from build123d import *

# Parameters (mm, degrees)
SKETCH_W        = 61
SKETCH_H        = 50
PAD_DEPTH       = 40
SKETCH001_W     = 58
SKETCH001_H     = 47
POCKET_DEPTH    = 23
SKETCH002_W     = 56
SKETCH002_H     = 45
POCKET001_DEPTH = 16
SKETCH003_W     = 1
SKETCH003_H     = 45
PAD001_DEPTH    = 3
SKETCH004_W     = 4
SKETCH004_H     = 11
POCKET002_DEPTH = 5
SKETCH005_W     = 5.5
SKETCH005_H     = 15.5
POCKET003_DEPTH = 23
SKETCH006_W     = 59
SKETCH006_H     = 48
POCKET004_DEPTH = 1
SKETCH007_W     = 2.5
SKETCH007_H     = 3.5
POCKET005_DEPTH = 23
SKETCH009_W     = 10
SKETCH009_H     = 5
POCKET006_DEPTH = 5
PAD002_DEPTH    = 2
SKETCH011_W     = 8
SKETCH011_H     = 4.5
POCKET007_DEPTH = 5
SKETCH012_W     = 15.5
SKETCH012_H     = 6
POCKET008_DEPTH = 5
SKETCH013_W     = 9
SKETCH013_H     = 1
POCKET009_DEPTH = 3
SKETCH014_W     = 1
SKETCH014_H     = 4.5
POCKET010_DEPTH = 5
SKETCH015_W     = 9
SKETCH015_H     = 0.5
POCKET011_DEPTH = 5
SKETCH016_W     = 17.5
SKETCH016_H     = 1
POCKET012_DEPTH = 5
SKETCH017_W     = 2
SKETCH017_H     = 6
POCKET013_DEPTH = 5
SKETCH018_W     = 1
SKETCH018_H     = 11
POCKET014_DEPTH = 5
SKETCH019_W     = 12
SKETCH019_H     = 1.5
POCKET015_DEPTH = 5
SKETCH020_W     = 2
SKETCH020_H     = 5
POCKET016_DEPTH = 5
SKETCH021_R     = 2.692582
POCKET017_DEPTH = 5
SKETCH022_W     = 1
SKETCH022_H     = 45
PAD003_DEPTH    = 3
SKETCH023_W     = 41
SKETCH023_H     = 1
PAD004_DEPTH    = 3
SKETCH024_W     = 1
SKETCH024_H     = 45
POCKET018_DEPTH = 3


with BuildPart() as part:
    # Sketch → Pad (new body)
    with BuildSketch(Plane.XY):
        with Locations((30.5, 25)):
            Rectangle(SKETCH_W, SKETCH_H)
    extrude(amount=PAD_DEPTH)

    # Sketch001 (on Face6 of Pad) → Pocket (cut)
    with BuildSketch(Plane.XY.offset(40)):
        with Locations((30.5, 25)):
            Rectangle(SKETCH001_W, SKETCH001_H)
    extrude(amount=-POCKET_DEPTH, mode=Mode.SUBTRACT)

    # Sketch002 (on Face11 of Pocket) → Pocket001 (cut)
    with BuildSketch(Plane.XY.offset(17)):
        with Locations((30.5, 25)):
            Rectangle(SKETCH002_W, SKETCH002_H)
    extrude(amount=-POCKET001_DEPTH, mode=Mode.SUBTRACT)

    # Sketch003 (on Face16 of Pocket001) → Pad001 (join)
    with BuildSketch(Plane.XY.offset(1)):
        with Locations((45, 25)):
            Rectangle(SKETCH003_W, SKETCH003_H)
    extrude(amount=PAD001_DEPTH)

    # Sketch004 (on Face20 of Pad001) → Pocket002 (cut)
    with BuildSketch(Plane.XY.offset(1)):
        with Locations((5, 13)):
            Rectangle(SKETCH004_W, SKETCH004_H)
    extrude(amount=-POCKET002_DEPTH, mode=Mode.SUBTRACT)

    # Sketch005 (on Face5 of Pocket002) → Pocket003 (cut)
    with BuildSketch(Plane.XY.offset(40)):
        with Locations((58.25, 42.25)):
            Rectangle(SKETCH005_W, SKETCH005_H)
    extrude(amount=-POCKET003_DEPTH, mode=Mode.SUBTRACT)

    # Sketch006 (on Face5 of Pocket003) → Pocket004 (cut)
    with BuildSketch(Plane.XY.offset(40)):
        with Locations((30.5, 25)):
            Rectangle(SKETCH006_W, SKETCH006_H)
    extrude(amount=-POCKET004_DEPTH, mode=Mode.SUBTRACT)

    # Sketch007 (on Face5 of Pocket004) → Pocket005 (cut)
    with BuildSketch(Plane.XY.offset(40)):
        with Locations((59.75, 32.75)):
            Rectangle(SKETCH007_W, SKETCH007_H)
    extrude(amount=-POCKET005_DEPTH, mode=Mode.SUBTRACT)

    # Sketch009 (on Face1 of Pocket005) → Pocket006 (cut)
    with BuildSketch(Plane.XZ):
        with Locations((21, 23.5)):
            Rectangle(SKETCH009_W, SKETCH009_H)
    extrude(amount=-POCKET006_DEPTH, mode=Mode.SUBTRACT)

    # Sketch010 (on Face21 of Pocket006) → Pad002 (join)
    with BuildSketch(Plane.XY.offset(17)):
        Polygon((55.5, 50), (61, 50), (61, 31), (59.5, 31), (59.5, 48.5), (55.5, 48.5), align=None)
    extrude(amount=PAD002_DEPTH)

    # Sketch011 (on Face31 of Pad002) → Pocket007 (cut)
    with BuildSketch(Plane.YZ.offset(2.5)):
        with Locations((8, 9.75)):
            Rectangle(SKETCH011_W, SKETCH011_H)
    extrude(amount=-POCKET007_DEPTH, mode=Mode.SUBTRACT)

    # Sketch012 (on Face28 of Pocket007) → Pocket008 (cut)
    with BuildSketch(Plane.YZ.offset(2.5)):
        with Locations((29.25, 8)):
            Rectangle(SKETCH012_W, SKETCH012_H)
    extrude(amount=-POCKET008_DEPTH, mode=Mode.SUBTRACT)

    # Sketch013 (on Face2 of Pocket008) → Pocket009 (cut)
    with BuildSketch(Plane(origin=(0, 0, 0), x_dir=(0, -1, 0), z_dir=(-1, 0, 0))):
        with Locations((-8.5, 12.5)):
            Rectangle(SKETCH013_W, SKETCH013_H)
    extrude(amount=-POCKET009_DEPTH, mode=Mode.SUBTRACT)

    # Sketch014 (on Face2 of Pocket009) → Pocket010 (cut)
    with BuildSketch(Plane(origin=(0, 0, 0), x_dir=(0, -1, 0), z_dir=(-1, 0, 0))):
        with Locations((-12.5, 9.75)):
            Rectangle(SKETCH014_W, SKETCH014_H)
    extrude(amount=-POCKET010_DEPTH, mode=Mode.SUBTRACT)

    # Sketch015 (on Face2 of Pocket010) → Pocket011 (cut)
    with BuildSketch(Plane(origin=(0, 0, 0), x_dir=(0, -1, 0), z_dir=(-1, 0, 0))):
        with Locations((-8.5, 13.25)):
            Rectangle(SKETCH015_W, SKETCH015_H)
    extrude(amount=-POCKET011_DEPTH, mode=Mode.SUBTRACT)

    # Sketch016 (on Face2 of Pocket011) → Pocket012 (cut)
    with BuildSketch(Plane(origin=(0, 0, 0), x_dir=(0, -1, 0), z_dir=(-1, 0, 0))):
        with Locations((-30.25, 11.5)):
            Rectangle(SKETCH016_W, SKETCH016_H)
    extrude(amount=-POCKET012_DEPTH, mode=Mode.SUBTRACT)

    # Sketch017 (on Face2 of Pocket012) → Pocket013 (cut)
    with BuildSketch(Plane(origin=(0, 0, 0), x_dir=(0, -1, 0), z_dir=(-1, 0, 0))):
        with Locations((-38, 8)):
            Rectangle(SKETCH017_W, SKETCH017_H)
    extrude(amount=-POCKET013_DEPTH, mode=Mode.SUBTRACT)

    # Sketch018 (on Face3 of Pocket013) → Pocket014 (cut)
    with BuildSketch(Plane(origin=(0, 0, 0), x_dir=(1, 0, 0), z_dir=(0, 0, -1))):
        with Locations((7.5, -13)):
            Rectangle(SKETCH018_W, SKETCH018_H)
    extrude(amount=-POCKET014_DEPTH, mode=Mode.SUBTRACT)

    # Sketch019 (on Face1 of Pocket014) → Pocket015 (cut)
    with BuildSketch(Plane.XZ):
        with Locations((22, 26.75)):
            Rectangle(SKETCH019_W, SKETCH019_H)
    extrude(amount=-POCKET015_DEPTH, mode=Mode.SUBTRACT)

    # Sketch020 (on Face1 of Pocket015) → Pocket016 (cut)
    with BuildSketch(Plane.XZ):
        with Locations((27, 23.5)):
            Rectangle(SKETCH020_W, SKETCH020_H)
    extrude(amount=-POCKET016_DEPTH, mode=Mode.SUBTRACT)

    # Sketch021 (on Face5 of Pocket016) → Pocket017 (cut)
    with BuildSketch(Plane.YZ.offset(61)):
        with Locations((15.5, 33.5)):
            Circle(SKETCH021_R)
    extrude(amount=-POCKET017_DEPTH, mode=Mode.SUBTRACT)

    # Sketch022 (on Face47 of Pocket017) → Pad003 (join)
    with BuildSketch(Plane.XY.offset(1)):
        with Locations((44, 25)):
            Rectangle(SKETCH022_W, SKETCH022_H)
    extrude(amount=PAD003_DEPTH)

    # Sketch023 (on Face47 of Pad003) → Pad004 (join)
    with BuildSketch(Plane.XY.offset(1)):
        with Locations((23, 44)):
            Rectangle(SKETCH023_W, SKETCH023_H)
    extrude(amount=PAD004_DEPTH)

    # Sketch024 (on Face68 of Pad004) → Pocket018 (cut)
    with BuildSketch(Plane.XY.offset(4)):
        with Locations((45, 25)):
            Rectangle(SKETCH024_W, SKETCH024_H)
    extrude(amount=-POCKET018_DEPTH, mode=Mode.SUBTRACT)


solid = part.part
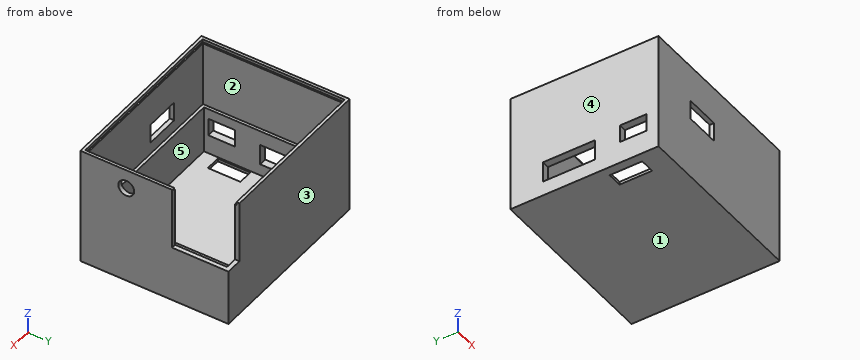
Could you check a few things on this model? Use its own coordinates, in mm. Face numbers are marked on the shaded views. A direction names the side the tool comes from. Coordinates: 2 decimals unless noted, no trailing zeros. Order: outer loops, then holes, each group sorted by start corner. A loop starts at its lowest first (then second) coordinate and runs counter-clockwise, first axis right, second up.
Q1. Will these pins go through, and if not, where does the flat tip stop? pin 1 (6 mm diameter, centred on x = 25.5, y = 7, fed in from -Z); pin 2 (3.5 mm diameter, centred on x = 14.5, y = 45.5, fed in from +Z); pin 3 (24 mm diameter, centred on x = 18.5, y = 16, fed in from +Z); pin 4 (0.8 mm diameter, centred on y = 49, z = 26, fed in from +X).
Q2. Please list where these lines run through material, in increasing order: L1, parallel to X at y = 18.5, z = 3.5; L2, parallel to Y at x = 29, z = 5.5; L3, parallel to X at y = 19.5, z = 21.
Q3. Suppose I cut it at A-A on z = 32.5. Please give me the cut outline in (x, y).
Q4. Which directions (+Z, -Z, +X, -X, +Y, -Y) give clear straight access to the entire face, cutting with the end or side of a thin tool? Please do the marked faces 4 and 5.
Q5. Suppose I cut it at C-C on x = 25. Please give me the cut outline in (y, z), and give its area (3 significant figures).
Q6. Thinking about a two-plate mould opening in Y: for the marked faces 1, 2 and 3, which applies, released by +Y, released by -Y, zero draft, split by the parting line, or undercut?
Q7. Suppose I cut it at D-D on z = 18. Please give me the cut outline in (x, y), and give its area (3 significant figures).
Q8. Suppose I cut it at B-B on y = 15.5. Please give me the cut outline in (x, z), and give its area (3 significant figures).
Answer:
1. pin 1: stops at z = 0
1. pin 2: stops at z = 4
1. pin 3: stops at z = 1
1. pin 4: stops at x = 55.5
2. L1: x = 0 to 2.5, 43.5 to 44.5, 58.5 to 61
2. L2: y = 0 to 2.5, 47.5 to 50
2. L3: x = 0 to 1.5, 59.5 to 61
3. outline: (0, 0) - (61, 0) - (61, 13) - (59.5, 13) - (59.5, 1.5) - (1.5, 1.5) - (1.5, 48.5) - (55.5, 48.5) - (55.5, 50) - (0, 50) - close; (59.5, 18) - (61, 18) - (61, 31) - (59.5, 31) - close
4. face 4: +Z, -Z, -X, +Y, -Y
4. face 5: +Z
5. outline: (0, 0) - (50, 0) - (50, 40) - (49, 40) - (49, 39) - (48.5, 39) - (48.5, 17) - (47.5, 17) - (47.5, 1) - (44.5, 1) - (44.5, 4) - (43.5, 4) - (43.5, 1) - (2.5, 1) - (2.5, 17) - (1.5, 17) - (1.5, 21) - (0, 21) - close; (0, 27.5) - (1.5, 27.5) - (1.5, 39) - (1, 39) - (1, 40) - (0, 40) - close
5. area: 191 mm2
6. face 1: zero draft
6. face 2: undercut
6. face 3: released by +Y
7. outline: (0, 0) - (61, 0) - (61, 50) - (0, 50) - close; hole (1.5, 1.5) - (59.5, 1.5) - (59.5, 48.5) - (1.5, 48.5) - close
7. area: 324 mm2
8. outline: (0, 0) - (3, 0) - (3, 1) - (2.5, 1) - (2.5, 17) - (1.5, 17) - (1.5, 39) - (1, 39) - (1, 40) - (0, 40) - close; (8, 0) - (61, 0) - (61, 30.81) - (59.5, 30.81) - (59.5, 17) - (58.5, 17) - (58.5, 1) - (44.5, 1) - (44.5, 4) - (43.5, 4) - (43.5, 1) - (8, 1) - close; (59.5, 36.19) - (61, 36.19) - (61, 40) - (60, 40) - (60, 39) - (59.5, 39) - close
8. area: 199 mm2
